```python
from build123d import *

# Parameters (mm, degrees)
SKETCH1_W           = 100
SKETCH1_H           = 36
BOSS_EXTRUDE1_DEPTH = 90
SHELL2_T            = -3
SKETCH3_W           = 15
SKETCH3_H           = 10.5
CUT_EXTRUDE3_DEPTH  = 10
SKETCH5_W           = 86
SKETCH5_H           = 2
CUT_EXTRUDE4_DEPTH  = 98
SKETCH6_R           = 7.5
CUT_EXTRUDE5_DEPTH  = 10


with BuildPart() as part:
    # Sketch1 → Boss-Extrude1 (new body)
    with BuildSketch(Plane.XY):
        with Locations((50, -18)):
            Rectangle(SKETCH1_W, SKETCH1_H)
    extrude(amount=BOSS_EXTRUDE1_DEPTH)

    # Shell2
    shell2_openings = [part.faces().sort_by_distance(p)[0] for p in [
        (50, 0, 45),
    ]]
    offset(amount=SHELL2_T, openings=shell2_openings, kind=Kind.INTERSECTION)

    # Sketch3 → Cut-Extrude3 (cut)
    with BuildSketch(Plane.XY.offset(90)):
        with Locations((81, -27.75)):
            Rectangle(SKETCH3_W, SKETCH3_H)
    extrude(amount=-CUT_EXTRUDE3_DEPTH, mode=Mode.SUBTRACT)

    # Sketch5 → Cut-Extrude4 (cut)
    with BuildSketch(Plane(origin=(100, 0, 0), x_dir=(0, 0, -1), z_dir=(1, 0, 0))):
        with Locations((-45, -3)):
            Rectangle(SKETCH5_W, SKETCH5_H)
    extrude(amount=-CUT_EXTRUDE4_DEPTH, mode=Mode.SUBTRACT)

    # Sketch6 → Cut-Extrude5 (cut)
    with BuildSketch(Plane(origin=(100, 0, 0), x_dir=(0, 0, -1), z_dir=(1, 0, 0))):
        with Locations((-45, -23.5)):
            Circle(SKETCH6_R)
    extrude(amount=-CUT_EXTRUDE5_DEPTH, mode=Mode.SUBTRACT)


solid = part.part
```
Model file for the job. Use its own axes, mm. A direction names the side the tool comes from. Coordinates: 2 decimals unless noted, no trailing zeros. Order: outer loops, then holes, each group sorted by start corner. A loop starts at its lowest first (then second) coordinate and runs counter-clockwise, first axis right, second up. Notation, with made-up numbers: (70.25, 81) - (129.25, 81) arc R24 cw to (129.25, 98) - close; hole circle Ø9 at (49.5, -16.75). An arc over 180 degrees is marked (long way). Return JSON: item names as keys, results as strings. Group by question number.
1) Probe line 1 (Y direction, x = 98.7, z = 45); line 2 (X direction, y = -12, z = 16.5); line 3 (Z direction, x = 78, y = -10.5). List the from-to ranges inside material, lowest first. Write a range as from..to.
2) Mould opens along Y. For faces 1 (the flat face through (98, -2, 45)), 2 (the flat face through (100, -14, 44)), 3 (the flat face through (49, -36, 44)) say: released by +Y, released by -Y, zero draft, split by the parting line, or undercut.
3) Saw through at A-A, the plane z = 20. Write the cut outline in (x, y).
4) Saw through at D-D, the plane y = -26.5. Write the cut outline in (x, z), plus the area to 3 significant figures.
5) Saw through at C-C, the plane x = 52.5. Write the cut outline in (y, z), plus the area to 3 significant figures.
6) Saw through at B-B, the plane z = 45. Write the cut outline in (x, y), plus the area to 3 significant figures.
7) Tool access for faces 4 (the flat face through (88.5, -28, 89)), 5 (the flat face through (0, -18, 44)), 6 (the flat face through (98, -4, 45)), 7 (the flat face through (49, -18, 87)): list every direction of +Z, -Z, +X, -X, +Y, -Y with a clear straight run to the whole face (end or side of a thin tool).
Values found:
{
 "1": {"line 1": "y = -36..-31, -16..-4, -2..0", "line 2": "x = 0..3, 97..100", "line 3": "z = 0..3, 87..90"},
 "2": {"face 1": "undercut", "face 2": "zero draft", "face 3": "released by -Y"},
 "3": {"outline": "(0, -36) - (100, -36) - (100, -4) - (97, -4) - (97, -33) - (3, -33) - (3, -4) - (2, -4) - (2, -2) - (3, -2) - (3, 0) - (0, 0) - close; (97, -2) - (100, -2) - (100, 0) - (97, 0) - close"},
 "4": {"outline": "(0, 0) - (100, 0) - (100, 38.13) - (97, 38.13) - (97, 3) - (3, 3) - (3, 87) - (73.5, 87) - (73.5, 90) - (0, 90) - close; (88.5, 87) - (97, 87) - (97, 51.87) - (100, 51.87) - (100, 90) - (88.5, 90) - close", "area": "1,020 mm²"},
 "5": {"outline": "(-36, 0) - (0, 0) - (0, 3) - (-2, 3) - (-2, 2) - (-4, 2) - (-4, 3) - (-33, 3) - (-33, 87) - (-4, 87) - (-4, 88) - (-2, 88) - (-2, 87) - (0, 87) - (0, 90) - (-36, 90) - close", "area": "464 mm²"},
 "6": {"outline": "(0, -36) - (100, -36) - (100, -31) - (97, -31) - (97, -33) - (3, -33) - (3, -4) - (2, -4) - (2, -2) - (3, -2) - (3, 0) - (0, 0) - close; (97, -16) - (100, -16) - (100, -4) - (97, -4) - close; (97, -2) - (100, -2) - (100, 0) - (97, 0) - close", "area": "445 mm²"},
 "7": {"face 4": "+Z", "face 5": "+Z, -Z, -X, +Y, -Y", "face 6": "+X", "face 7": "+Y"}
}
